Can you work these out from the model? Positions are in its coordinate system, mm. Give positions to 0.01 mm unless a question says otherwise; leave off trailing zeros. Loops run counter-clockwise (first coordinate to the right, second up) from the corner with the lowest first, then second, coordinate; pieces in that order, holes last. Notation, with made-up numbers: M 53,53.5 L 80,53.5 A17 cw 80,64.5 Z; hole C -19.75,75 d1. An arc over 180 degrees is marked long. Use CSV: the item, a comma, the result in double quotes.
from build123d import *

# Parameters (mm, degrees)
STOCK_HAMMERSAW_START                   = -149.225
STOCK_HAMMERSAW_MULTIBODY_1_OUTLINE_R   = 2.5527
STOCK_HAMMERSAW_MULTIBODY_1_OUTLINE_R_2 = 7.62
STOCK_HAMMERSAW_MULTIBODY_1_OUTLINE_R_3 = 2.54
STOCK_HAMMERSAW_MULTIBODY_1_DEPTH       = 9.525
FILLET1_R                               = 2.54
FILLET2_R                               = 3.175
FILLET3_R                               = 25.4
FILLET4_R                               = 2.54
CUT_EXTRUDE1_DEPTH                      = 201.10578904
CUT_EXTRUDE1_DEPTH_BACK                 = 201.10578904
SKETCH1_W                               = 1.5875
SKETCH1_H                               = 240.255072357


with BuildPart() as part:
    # Stock-HammerSaw Multibody-1: read off the stored shape, not the designer's step
    # Stock-HammerSaw Multibody-1 outline → Stock-HammerSaw Multibody-1 (new body)
    with BuildSketch(Plane.YZ.offset(STOCK_HAMMERSAW_START)):
        with BuildLine():
            Line((9.525, 42.121134838), (9.525, -171.391646474))
            ThreePointArc((9.525, -171.391646474), (14.605, -176.471646474), (9.525, -181.551646474))
            Line((9.525, -181.551646474), (9.525, -195.537119935))
            Line((9.525, -195.537119935), (50.8, -160.903282658))
            Line((50.8, -160.903282658), (53.975, -66.675))
            Line((53.975, -66.675), (53.975, 42.121134838))
            ThreePointArc((53.975, 42.121134838), (31.75, 47.625), (9.525, 42.121134838))
        make_face()
        with Locations((17.944382949, -182.255416592)):
            Circle(STOCK_HAMMERSAW_MULTIBODY_1_OUTLINE_R, mode=Mode.SUBTRACT)
        with Locations((28.88924293, -173.071588618)):
            Circle(STOCK_HAMMERSAW_MULTIBODY_1_OUTLINE_R, mode=Mode.SUBTRACT)
        with Locations((25.4, -139.326770285)):
            Circle(STOCK_HAMMERSAW_MULTIBODY_1_OUTLINE_R_2, mode=Mode.SUBTRACT)
        with Locations((27.413358223, -95.151227202)):
            Circle(STOCK_HAMMERSAW_MULTIBODY_1_OUTLINE_R, mode=Mode.SUBTRACT)
        with Locations((19.05, -61.986201926)):
            Circle(STOCK_HAMMERSAW_MULTIBODY_1_OUTLINE_R, mode=Mode.SUBTRACT)
        with Locations((29.726233837, -44.403906028)):
            Circle(STOCK_HAMMERSAW_MULTIBODY_1_OUTLINE_R, mode=Mode.SUBTRACT)
        with Locations((14.2875, 37.399020291)):
            Circle(STOCK_HAMMERSAW_MULTIBODY_1_OUTLINE_R_3, mode=Mode.SUBTRACT)
        with Locations((25.761047521, 40.838193804)):
            Circle(STOCK_HAMMERSAW_MULTIBODY_1_OUTLINE_R_3, mode=Mode.SUBTRACT)
        with Locations((44.45, -61.986201926)):
            Circle(STOCK_HAMMERSAW_MULTIBODY_1_OUTLINE_R, mode=Mode.SUBTRACT)
        with Locations((31.75, 0)):
            Circle(STOCK_HAMMERSAW_MULTIBODY_1_OUTLINE_R_2, mode=Mode.SUBTRACT)
        with Locations((37.738952479, 40.838193804)):
            Circle(STOCK_HAMMERSAW_MULTIBODY_1_OUTLINE_R_3, mode=Mode.SUBTRACT)
        with Locations((49.2125, 37.399020291)):
            Circle(STOCK_HAMMERSAW_MULTIBODY_1_OUTLINE_R_3, mode=Mode.SUBTRACT)
    extrude(amount=STOCK_HAMMERSAW_MULTIBODY_1_DEPTH)


with BuildPart() as part_1:
    # Body-Move/Copy2: read off the stored shape, not the designer's step
    # Body-Move/Copy2: moved
    add(part.part.moved(Location((144.4625, 0, 0))))

    # Fillet1
    fillet1_edges = [part_1.edges().sort_by_distance(p)[0] for p in [
        (0, 9.525, -195.537119935),
    ]]
    fillet(fillet1_edges, radius=FILLET1_R)

    # Fillet2
    fillet2_edges = [part_1.edges().sort_by_distance(p)[0] for p in [
        (0, 53.975, 42.121134838),
        (0, 9.525, 42.121134838),
    ]]
    fillet(fillet2_edges, radius=FILLET2_R)

    # Fillet3
    # the kernel refuses this fillet: 25.4 mm, written as the material it takes off along each edge
    with BuildSketch(Plane(origin=(-33.08112114, 50.8, -160.903282658), x_dir=(0, -0.7660444431175363, -0.6427876096882575), z_dir=(1, 0, 0))) as fillet3_piece_1:
        with BuildLine():
            CenterArc((FILLET3_R * 0.445962537632, -FILLET3_R), FILLET3_R, 90, 48.070162195)
            Line((-FILLET3_R * 0.2980011219, -FILLET3_R * 0.33177992151), (0, 0))
            Line((0, 0), (FILLET3_R * 0.445962537632, 0))
        make_face()
    extrude(amount=66.162242279, mode=Mode.SUBTRACT)
    with BuildSketch(Plane(origin=(-5.832005366, 53.975, -66.675), x_dir=(0, 0, 1), z_dir=(1, 0, 0))) as fillet3_piece_2:
        with BuildLine():
            CenterArc((FILLET3_R * 0.0168426041932, FILLET3_R), FILLET3_R, 268.070162195, 1.929837805)
            Line((-FILLET3_R * 0.0168330513083, FILLET3_R * 0.000567185736557), (0, 0))
            Line((0, 0), (FILLET3_R * 0.0168426041932, 0))
        make_face()
    extrude(amount=11.664010733, mode=Mode.SUBTRACT)

    # Fillet4
    fillet4_edges = [part_1.edges().sort_by_distance(p)[0] for p in [
        (0, 9.525, -181.551646474),
        (0, 9.525, -171.391646474),
    ]]
    fillet(fillet4_edges, radius=FILLET4_R)

    # Sketch1 → Cut-Extrude1 (cut, two sides: drawn at the far end of the back side and taken through both)
    with BuildSketch(Plane(origin=(0, 0, 0), x_dir=(1, 0, 0), z_dir=(0, 1, 0)).offset(-CUT_EXTRUDE1_DEPTH_BACK)):
        with Locations((-3.96875, 72.502536179)):
            Rectangle(SKETCH1_W, SKETCH1_H)
        with Locations((3.96875, 72.502536179)):
            Rectangle(SKETCH1_W, SKETCH1_H)
    extrude(amount=CUT_EXTRUDE1_DEPTH + CUT_EXTRUDE1_DEPTH_BACK, mode=Mode.SUBTRACT)


solid = part_1.part
Q1. Please list where these lines run through material, in increasing order: L1, parallel to Z at x = -1.25, y = 31.75 (3 decimals); L2, parallel to Z at x = -0.5, y = 26; L3, parallel to Z at x = -1, y = 25.4. Write a range as from..to.
Model answer:
L1,"-176.888..-143.539, -135.115..-45.96, -42.848..-7.62, 7.62..47.625"
L2,"-181.71..-146.92, -131.73..-97.28, -93.03..-5, 5..38.31, 43.37..47.28"
L3,"-182.22..-146.95, -131.71..-96.72, -93.58..-4.21, 4.21..38.32, 43.35..47.2"
Q2. If we mould it in two halves opening along Z, with no side actions, what happens to faces 1 (the flat face through (3.175, 31, -71)), 2 (the cylindrical face through (-0.044, 48.566, -159.981)), 3 (the cylindrical face through (-0.044, 23.745, 39.293)), 4 (the cylindrical face through (-0.04, 43.9, -64.48))? For each: released by +Z, released by -Z, zero draft, split by the parting line, or undercut.
Model answer:
face 1,"zero draft"
face 2,"released by -Z"
face 3,"undercut"
face 4,"undercut"
Q3. I want a section at B-B, the plane z = 4. Please give me the cut outline in (x, y) (3 decimals).
Model answer:
outline,"M -3.175,9.525 L 3.175,9.525 L 3.175,25.264 L -3.175,25.264 Z; M -3.175,38.236 L 3.175,38.236 L 3.175,53.975 L -3.175,53.975 Z"
Q4. I want a section at C-C, the plane x = -0.75. State how many separate pieces and enclosed holes the cut face has, then the cut area to 3 significant figures.
Model answer:
separate pieces,"1"
enclosed holes,"12"
area,"9,120 mm2"
Q5. I want a section at A-A, the plane y = 44.45. Please give me the cut outline in (x, z) (1 decimal).
Model answer:
outline,"M -3.2,-166 L 3.2,-166 L 3.2,-64.5 L -3.2,-64.5 Z; M -3.2,-59.4 L 3.2,-59.4 L 3.2,45.9 L -3.2,45.9 Z"
